```python
from build123d import *

# Parameters (mm, degrees)
SKETCH1_W           = 85
SKETCH1_H           = 10
BOSS_EXTRUDE1_DEPTH = 10
SKETCH2_R           = 1.4
CUT_EXTRUDE1_DEPTH  = 10
SKETCH3_W           = 5
SKETCH3_H           = 10
BOSS_EXTRUDE2_DEPTH = 32
SKETCH4_R           = 2.95
BOSS_EXTRUDE3_DEPTH = 4


with BuildPart() as part:
    # Sketch1 → Boss-Extrude1 (new body)
    with BuildSketch(Plane(origin=(0, 0, 0), x_dir=(1, 0, 0), z_dir=(0, 1, 0))):
        Rectangle(SKETCH1_W, SKETCH1_H)
    extrude(amount=BOSS_EXTRUDE1_DEPTH)

    # Sketch2 → Cut-Extrude1 (cut)
    with BuildSketch(Plane(origin=(0, 10, 0), x_dir=(1, 0, 0), z_dir=(0, 1, 0))):
        with Locations(Location((35, 0, 0), (0, 0, 270))):
            Circle(SKETCH2_R)
        with Locations(Location((20, 0, 0), (0, 0, 270))):
            Circle(SKETCH2_R)
    extrude(amount=-CUT_EXTRUDE1_DEPTH, mode=Mode.SUBTRACT)

    # Sketch3 → Boss-Extrude2 (add)
    with BuildSketch(Plane.XY.offset(5)):
        with Locations((-40, 5)):
            Rectangle(SKETCH3_W, SKETCH3_H)
    extrude(amount=BOSS_EXTRUDE2_DEPTH)

    # Sketch4 → Boss-Extrude3 (add)
    with BuildSketch(Plane(origin=(-37.5, 0, 0), x_dir=(0, 0, -1), z_dir=(1, 0, 0))):
        with Locations(Location((-31.75, 5, 0), (0, 0, 180))):
            Circle(SKETCH4_R)
    extrude(amount=BOSS_EXTRUDE3_DEPTH)


solid = part.part
```
Geometry check sheet. Reference: the model listing, model coordinates, mm. A direction names the side the tool comes from. Give positions to 0.01 mm unless a question says otherwise; leave off trailing zeros. Write each loop counter-clockwise with the first axis right and the second up, starting at its lowest first coordinate (ties: lowest second). Pieces come first, ordered by that corner, then holes. Notation, with made-up numbers: (-14, 38) -> (1, 38) arc R5 cw to (1, 46) -> close; hole circle Ø10 at (8, 25). An arc over 180 degrees is marked (long way). One line per question, with ' | ' between items.
Item 1: Sectioned sample at C-C, the plane z = 0. Record the boundary of the cut face in (x, y).
Determined:
outline: (-42.5, 0) -> (18.6, 0) -> (18.6, 10) -> (-42.5, 10) -> close; (21.4, 0) -> (33.6, 0) -> (33.6, 10) -> (21.4, 10) -> close; (36.4, 0) -> (42.5, 0) -> (42.5, 10) -> (36.4, 10) -> close
Item 2: Sectioned sample at A-A, the plane y = 5. Record the boundary of the cut face in (x, z), plus the area to 3 significant figures.
Determined:
outline: (-42.5, -5) -> (42.5, -5) -> (42.5, 5) -> (-37.5, 5) -> (-37.5, 28.8) -> (-33.5, 28.8) -> (-33.5, 34.7) -> (-37.5, 34.7) -> (-37.5, 37) -> (-42.5, 37) -> close; hole circle Ø2.8 at (20, 0); hole circle Ø2.8 at (35, 0) | area: 1,020 mm^2
Item 3: Access from +Z, -Z, +X, -X, +Y, -Y to the whole of each face (thin tool, end or side, straight path). Record for faces 4 (the flat face through (42.5, 5, 0)), 5 (the flat face through (-33.5, 5, 32)), 6 (the cylindrical face through (-35.528, 4.114, 34.564)).
Determined:
face 4: +Z, -Z, +X, +Y, -Y | face 5: +Z, +X, +Y, -Y | face 6: +X
Item 4: Sectioned sample at D-D, the plane z = 31.75. Record the boundary of the cut face in (x, y).
Determined:
outline: (-42.5, 0) -> (-37.5, 0) -> (-37.5, 2.05) -> (-33.5, 2.05) -> (-33.5, 7.95) -> (-37.5, 7.95) -> (-37.5, 10) -> (-42.5, 10) -> close
Item 5: Scan lines: line 1 along X through (y, z) = (3.75, 0); line 2 along X through (y, z) = (1, -1); line 3 along Z through (x, y) = (14, 6.75). Record each from-to range of solid material in increasing order.
Determined:
line 1: -42.5 to 18.6, 21.4 to 33.6, 36.4 to 42.5 | line 2: -42.5 to 19.02, 20.98 to 34.02, 35.98 to 42.5 | line 3: -5 to 5
Item 6: Sectioned sample at B-B, the plane x = 35. Record the boundary of the cut face in (y, z), plus the area to 3 significant figures.
Determined:
outline: (0, -5) -> (10, -5) -> (10, -1.4) -> (0, -1.4) -> close; (0, 1.4) -> (10, 1.4) -> (10, 5) -> (0, 5) -> close | area: 72.0 mm^2
Item 7: Draft check along X on faces 1 (the cylindrical face through (18.633, 5.07, -0.303)), 2 (the flat face through (-10, 0, 2)), 3 (the flat face through (-37.5, 5, 21)). Enter one of: released by +X, released by -X, zero draft, split by the parting line, or undercut.
Determined:
face 1: undercut | face 2: zero draft | face 3: released by +X
